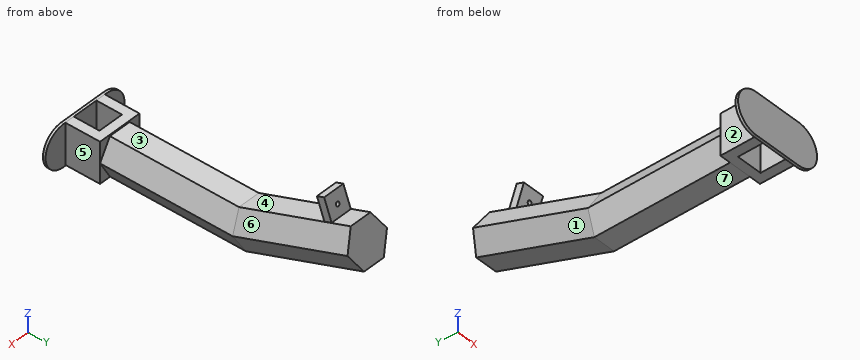
Autodesk Inventor part; units mm, degrees
sketch "Sketch1" plane through (0, 0, 0) normal (0, 1, 0) x (-1, 0, 0)
  line L0 (0, 0) -> (17.5, 0)
  line L1 (17.5, 0) -> (8.75, -15.1554)
  line L2 (8.75, -15.1554) -> (-8.75, -15.1554)
  line L3 (-8.75, -15.1554) -> (-17.5, 0)
  line L4 (-17.5, 0) -> (-8.75, 15.1554)
  line L5 (-8.75, 15.1554) -> (8.75, 15.1554)
  line L6 (8.75, 15.1554) -> (17.5, 0)
  dimension "d1" = 17.5
sketch "Sketch3" plane through (0, 0, 0) normal (1, 0, 0) x (0, 1, 0)
  line L0 (0, 0) -> (130, 0)
  line L1 (130, 0) -> (219.2708, 32.4919)
  dimension "d5" = 130
  dimension "d6" = 95
  dimension "d7" = 160
sweep "Sweep1" add profiles "Sketch1" path "Sketch3"
sketch "Sketch4" plane through (-8.75, 127.3277, 15.1554) normal (0, -0.3420201, 0.9396926) x (1, 0, 0)
  line L0 (0, 92.3277) -> (17.5, 92.3277)
  line L1 (8.75, 92.3277) -> (8.75, 76.3277)
  line L2 (8.75, 76.3277) -> (17.25, 76.3277)
  line L3 (17.5, 0) -> (17.5, 92.3277)
  line L4 (17.25, 76.3277) -> (17.25, 70.3277)
  line L5 (17.25, 70.3277) -> (0.25, 70.3277)
  line L6 (0, 0) -> (0, 92.3277)
  line L7 (0.25, 70.3277) -> (0.25, 76.3277)
  line L8 (0.25, 76.3277) -> (8.75, 76.3277)
  point P0 (8.75, -124.8324)
  dimension "d10" = 16
  dimension "d11" = 8.5
  dimension "d12" = 6
  dimension "d13" = 17
extrude "Extrusion1" add sketch "Sketch4" along normal blind 17
sketch "Sketch5" plane through (-8.5, 199.0522, 41.2611) normal (0, 0.9396926, 0.3420201) x (1, 0, 0)
  line L0 (17, 0) -> (0, 0)
  line L1 (8.5, 0) -> (8.5, -8)
  circle A0 centre (8.5, -8) radius 2.5
  point P0 (8.5, -29.3072)
  dimension "d16" = 8
  dimension "d17" = 5
hole "Hole1" at (0, 196.3161, 48.7786) direction (0, -0.9396926, -0.3420201) diameter 3 depth 10.077 tip angle 118
sketch "Sketch6" plane through (0, 0, 0) normal (0, 1, 0) x (-1, 0, 0)
  line L0 (17.5, 0) -> (8.75, 15.1554)
  line L1 (17.5, 0) -> (17.5, -15.4226)
  line L2 (17.5, -15.4226) -> (-17.5, -15.4226)
  line L3 (-17.5, -15.4226) -> (-17.5, 16.246)
  line L4 (-17.5, 0) -> (-17.5, 32.4919)
  line L5 (17.5, 0) -> (17.5, 32.4919)
  line L6 (17.5, 16.246) -> (-17.5, 16.246)
  line L7 (17.5, 16.246) -> (17.5, 0)
  point P0 (0, 0)
extrude "Extrusion2" add sketch "Sketch6" along normal blind 27
sketch "Sketch7" plane through (-17.5, 0, 16.246) normal (0, 0, 1) x (1, 0, 0)
  line L0 (17.5, 0) -> (7.5, 0)
  line L1 (35, 0) -> (0, 0)
  line L2 (7.5, 0) -> (27.5, 0)
  line L3 (7.5, 0) -> (7.5, 20)
  line L4 (7.5, 20) -> (27.5, 20)
  line L5 (27.5, 20) -> (27.5, 0)
  dimension "d27" = 10
  dimension "d28" = 20
  dimension "d29" = 20
extrude "Extrusion3" cut sketch "Sketch7" against normal blind 50
sketch "Sketch8" plane through (0, 0, 0) normal (0, 1, 0) x (-1, 0, 0)
  line L0 (0, 0) -> (-35, 0)
  line L1 (-35, 0) -> (35, 0) construction
  line L2 (-18.8264, -16.1736) -> (18.8264, -16.1736)
  line L3 (18.8264, 16.1736) -> (-18.8264, 16.1736)
  arc A0 (-18.8264, 16.1736) -> (-18.8264, -16.1736) centre (-18.8264, 0) ccw
  arc A1 (18.8264, -16.1736) -> (18.8264, 16.1736) centre (18.8264, 0) ccw
  dimension "d32" = 35
  dimension "d33" = 70
extrude "Extrusion4" add sketch "Sketch8" against normal blind 2
properties part number "Kamerahalter_II"
The listing builds one solid part. Answer for the finished solid, in the listing's coordinates (mm). Face numbers are marked on the shaded views. A direction names the side the tool comes from. Round coordinates to 2 decimals unless told otherwise and drop trailing zeros. Write each loop counter-clockwise with the first axis right and the second up, starting at its lowest first coordinate (ties: lowest second). Pieces come first, ordered by that corner, then holes. Notation, with made-up numbers: (23.25, -4) -> (65.25, -4) arc R17 ccw to (65.25, 16) -> close; hole circle Ø3 at (88.5, 19). An arc over 180 degrees is marked (long way). Write item = value, one per line.
1) For a pull along Y with two mould halves and no side action, classify the marked faces 1, 2, 3 and 4 as released by +Y, released by -Y, zero draft, split by the parting line, or undercut.
Check values:
face_1 = released by +Y
face_2 = zero draft
face_3 = undercut
face_4 = undercut
2) Given pin 1 (5 mm diameter, centred on x = 0.5, y = 82, fed in from -Z); pin 2 (12.5 mm diameter, centred on y = 192, z = 50, fed in from +X); pin 3 (2 mm diameter, centred on x = -8.5, y = -0.5, fed in from +Z), each flat-ended and moving along its own axis, determine where each tip first touches the part or whether it passes through.
Check values:
pin_1 = -15.16
pin_2 = 8.5
pin_3 = 16.17
3) Section D-D on x = -14.5 is taken. Write down the section's boundary in (y, z), plus the area to 3 significant figures.
Check values:
outline = (-2, -16.17) -> (0, -16.17) -> (0, -15.42) -> (27, -15.42) -> (27, -5.2) -> (130.92, -5.2) -> (221.05, 27.61) -> (217.49, 37.37) -> (129.08, 5.2) -> (27, 5.2) -> (27, 16.25) -> (0, 16.25) -> (0, 16.17) -> (-2, 16.17) -> close
area = 2,980 mm²
4) Which of the six approach directions +Z, -Z, +X, -X, +Y, -Y give full straight-line access (tool end or side, diameter ignored) to the marked faces 5, 6 and 7?
Check values:
face_5 = +Z, -Z, +X, +Y
face_6 = +Z, +X
face_7 = -Z, +X, -X, +Y
5) Straight lines are drawn through the part: line 1 along Z through (x, y) = (-1, 111); line 2 along Y through (x, z) = (-31.5, 7); line 3 along X through (y, z) = (58, 4). For each, find the intervals that lie inside material, in ascending order. Write a range as [from, to].
Check values:
line_1 = [-15.16, 15.16]
line_2 = [-2, 0]
line_3 = [-15.19, 15.19]
6) Section B-B on z = -8.5 is taken. Write down the section's boundary in (x, y).
Check values:
outline = (-32.59, -2) -> (32.59, -2) -> (32.59, 0) -> (17.5, 0) -> (17.5, 27) -> (12.59, 27) -> (12.59, 131.5) -> (8.75, 150.96) -> (-8.75, 150.96) -> (-12.59, 131.5) -> (-12.59, 27) -> (-17.5, 27) -> (-17.5, 0) -> (-32.59, 0) -> close; hole (-10, 0) -> (10, 0) -> (10, 20) -> (-10, 20) -> close
7) Section A-A on y = 12.5 is taken. Write down the section's boundary in (x, z), plus the area to 3 significant figures.
Check values:
outline = (-17.5, -15.42) -> (-10, -15.42) -> (-10, 16.25) -> (-17.5, 16.25) -> close; (10, -15.42) -> (17.5, -15.42) -> (17.5, 16.25) -> (10, 16.25) -> close
area = 475 mm²
8) Section C-C on y = 160.5 is taken. Write down the section's boundary in (x, z), plus the area to 3 significant figures.
Check values:
outline = (-17.5, 11.1) -> (-8.75, -5.03) -> (8.75, -5.03) -> (17.5, 11.1) -> (8.75, 27.23) -> (-8.75, 27.23) -> close
area = 847 mm²
